```python
from build123d import *

# Parameters (mm, degrees)
SKETCH3_R               = 50.7
SKETCH3_R_2             = 40.700000007
BOSS_EXTRUDE1_DEPTH     = 20
CUT_EXTRUDE1_REACH      = 117.119
CUT_EXTRUDE1_END_RADIUS = 40.700000007
SKETCH5_R               = 2.5
CIRPATTERN1_COUNT       = 8


with BuildPart() as part:
    # Sketch3 → Boss-Extrude1 (new body)
    with BuildSketch(Plane(origin=(0, 0, 0), x_dir=(1, 0, 0), z_dir=(0, 1, 0))):
        with Locations(Location((0, 0, 0), (0, 0, 270))):
            Circle(SKETCH3_R)
        with Locations(Location((0, 0, 0), (0, 0, 270))):
            Circle(SKETCH3_R_2, mode=Mode.SUBTRACT)
    extrude(amount=BOSS_EXTRUDE1_DEPTH)

    # Cut-Extrude1: up to this cylinder (the profile starts outside it)
    cut_extrude1_end = Plane(origin=(0, 10, 0), z_dir=(0, -1, 0)) * Cylinder(CUT_EXTRUDE1_END_RADIUS, 316.638000014, mode=Mode.PRIVATE)
    # Sketch5 → Cut-Extrude1 (cut, up to the surface)
    with BuildSketch(Plane(origin=(50.7, 0, 0), x_dir=(0, 0, -1), z_dir=(1, 0, 0)), mode=Mode.PRIVATE) as cut_extrude1_sk1:
        with Locations((0, 10)):
            Circle(SKETCH5_R)
    cut_extrude1_tool1 = extrude(cut_extrude1_sk1.sketch, amount=-CUT_EXTRUDE1_REACH, mode=Mode.PRIVATE) - cut_extrude1_end
    cut_extrude1 = cut_extrude1_tool1.solids().sort_by_distance((50.7, 10, 0))[0]
    add(cut_extrude1, mode=Mode.SUBTRACT)

    # CirPattern1: Cut-Extrude1 ×8 about axis
    cirpattern1_axis = Axis((0, 20, 0), (0, -1, 0))
    for i in range(1, CIRPATTERN1_COUNT):
        add(cut_extrude1.rotate(cirpattern1_axis, i * 360 / CIRPATTERN1_COUNT), mode=Mode.SUBTRACT)


solid = part.part
```
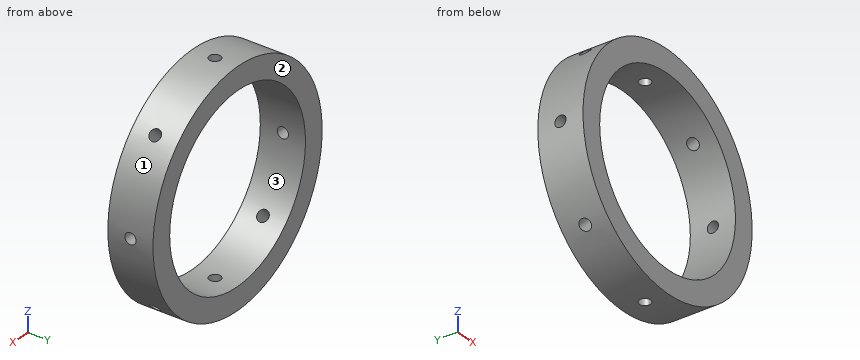
Check sheet for the modelled part. Datum: model origin and axes. Units: mm. Face numbers are marked on the shaded views. Coordinates: 2 decimals unless noted, no trailing zeros. Write each loop counter-clockwise with the first axis right and the second up, starting at its lowest first coordinate (ties: lowest second). Pieces come first, ordered by that corner, then holes. Notation, with made-up numbers: M -22.75,56.25 L -3.75,56.25 A21 cw -3.75,73.25 Z; hole C 65.5,74.5 d7. An arc over 180 degrees is marked long. Write item = value, one per line. Start each with the question number.
1. Sectioned sample at C-C (y = 10). State how many separate pieces and enclosed holes the cut face has, then the cut area to 3 significant figures.
2. Thickness scan on probe 1 along Y at (x, z) = (-45, 0); probe 2 along X at (y, z) = (7.25, -6.5); probe 3 along X at (y, z) = (5.75, 20.5). Record the ranges inside material, lowest first.
3. Sectioned sample at A-A (x = 0). Record the cut outline in (y, z).
4. Go/stop test with flat-tipped pins: pin 1 (8 mm diameter, centred on y = 17.5, z = 19.5, fed in from +X); pin 2 (4 mm diameter, centred on x = 34.5, y = 8, fed in from +Z); pin 3 (3 mm diameter, centred on y = 17.5, z = 35, fed in from -X); pin 4 (4.5 mm diameter, centred on y = 10, z = 0, fed in from +X). Record where each tip stops, or that it passes through.
5. Sectioned sample at D-D (y = 18.25). Record the cut outline in (x, z), then the cut area to 3 significant figures.
6. Sectioned sample at B-B (z = 0). Record the cut outline in (x, y), then the cut area to 3 significant figures.
7. Mould release check, pull along Z, two halves, no side actions. Record for the marked faces 1, 2 and 3: pulls with the +Z half, pulls with the -Z half, needs draft (parallel to the pull), parting line crosses it, or undercut.
The answers:
q1.separate_pieces = 8
q1.enclosed_holes = 0
q1.area = 2,470 mm²
q2.probe_1 = 0 to 7.5, 12.5 to 20
q2.probe_2 = -50.28 to -40.18, 40.18 to 50.28
q2.probe_3 = -46.37 to -35.16, 35.16 to 46.37
q3.outline = M 0,-50.7 L 7.5,-50.7 L 7.5,-40.7 L 0,-40.7 Z; M 0,40.7 L 7.5,40.7 L 7.5,50.7 L 0,50.7 Z; M 12.5,-50.7 L 20,-50.7 L 20,-40.7 L 12.5,-40.7 Z; M 12.5,40.7 L 20,40.7 L 20,50.7 L 12.5,50.7 Z
q4.pin_1 = 48.27
q4.pin_2 = 38.91
q4.pin_3 = -38.06
q4.pin_4 = through
q5.outline = C 0,0 d101.4; hole C 0,0 d81.4
q5.area = 2,870 mm²
q6.outline = M -50.7,0 L -40.7,0 L -40.7,7.5 L -50.7,7.5 Z; M -50.7,12.5 L -40.7,12.5 L -40.7,20 L -50.7,20 Z; M 40.7,0 L 50.7,0 L 50.7,7.5 L 40.7,7.5 Z; M 40.7,12.5 L 50.7,12.5 L 50.7,20 L 40.7,20 Z
q6.area = 300 mm²
q7.face_1 = parting line crosses it
q7.face_2 = needs draft
q7.face_3 = undercut
